Print and shaded views of the part. All mm, measured from the part's lowest x, y and z. Give positions to 0.01 mm unless a question says otherwise; leave off trailing zeros. Write each loop counter-clockwise with the first axis right and the second up, starting at its lowest first coordinate (ties: lowest second). Pieces come first, ordered by that corner, then holes. Notation, with made-up numbers: M -26,-28 L 20,-28 A11 ccw 20,-9 Z; hole C 69,78.25 d11. An arc over 180 degrees is marked long. One line per question, with ' | ' between items. Start each with the question number.
1. Wall check: L1, parallel to X at y = 11.5, z = 5; L2, parallel to X at y = 9.75, z = 6 (1 decimal); L3, parallel to Y at x = 41, z = 2.5 (1 decimal). Give the ranges that are in metal, low to high.
2. Cut at D-D, the plane x = 8.5. Write the cut outline in (y, z) (1 decimal), then the cut area to 3 significant figures.
3. Cut at B-B, the plane y = 15.25. Write the cut outline in (x, z) (1 decimal).
4. Cut at C-C, the plane x = 42.5. Write the cut outline in (y, z).
5. Flat gauge pins, fed straight in: pin 1 (4 mm diameter, centred on x = 7.5, z = 4, fed in from -Y); pin 2 (2 mm diameter, centred on y = 4, z = 4, fed in from +X). Where does each tip first touch, or does it go through?
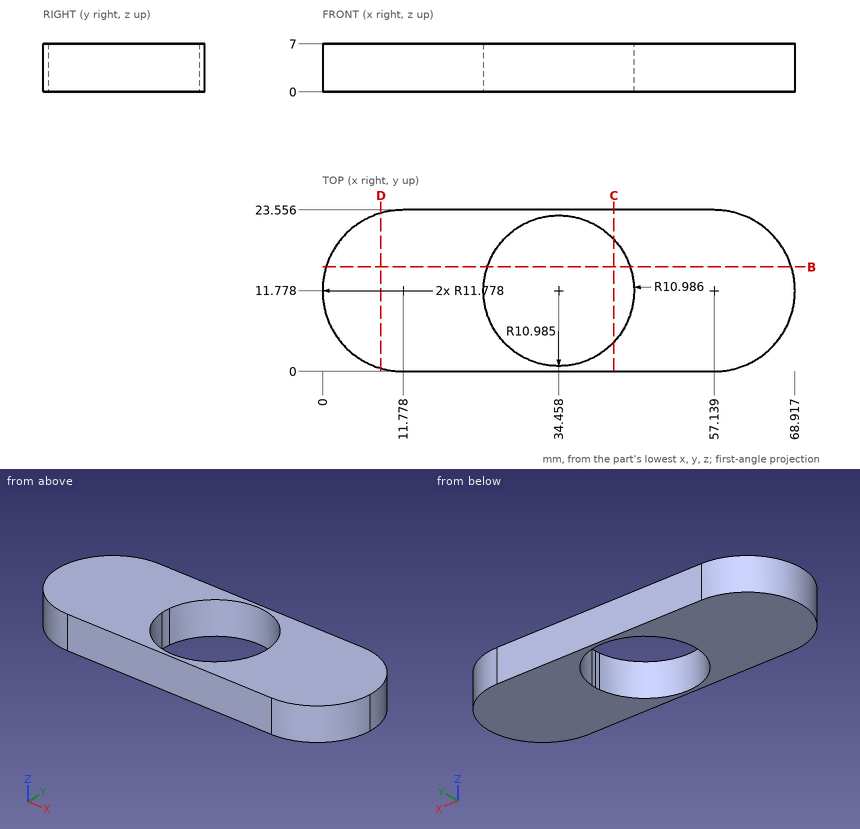
Here are the results:
1) L1: 0 to 23.48, 45.44 to 68.91 | L2: 0.2 to 23.7, 45.3 to 68.7 | L3: 0 to 3, 20.6 to 23.6
2) outline: M 0.5,0 L 23.1,0 L 23.1,7 L 0.5,7 Z | area: 158 mm^2
3) outline: M 0.5,0 L 24,0 L 24,7 L 0.5,7 Z; M 44.9,0 L 68.4,0 L 68.4,7 L 44.9,7 Z
4) outline: M 0,0 L 4.29,0 L 4.29,7 L 0,7 Z; M 19.26,0 L 23.56,0 L 23.56,7 L 19.26,7 Z
5) pin 1: y = 0.22 | pin 2: x = 66.77
